CAD build for the part. Positions are in the model's coordinates, mm. A direction names the side the tool comes from. Round coordinates to 2 decimals unless told otherwise and drop trailing zeros. Order: outer loops, then holes, each group sorted by start corner. A loop starts at its lowest first (then second) coordinate and runs counter-clockwise, first axis right, second up. Notation, with made-up numbers: M 51,15.5 L 68,15.5 A20 ccw 68,24.5 Z; hole C 7,26 d6. An arc over 180 degrees is marked long. Put each result on its own line as item: value.
```python
from build123d import *

# Parameters (mm, degrees)
F0_R     = 2
F1_DEPTH = 5
F2_R     = 3
F3_DEPTH = 10
F4_R     = 1.3
F5_DEPTH = 10


with BuildPart() as f1:
    # F0 (on Front) → F1 (new body)
    with BuildSketch(Plane.XZ):
        with BuildLine():
            Line((-2, 3.338963), (-2, 12.338963))
            ThreePointArc((-2, 12.338963), (-10.825318, 6.25), (-11.685855, -4.437431))
            Line((-11.685855, -4.437431), (-3.891627, 0.062569))
            Line((-3.891627, 0.062569), (-1.891627, -3.401532))
            Line((-1.891627, -3.401532), (-9.685855, -7.901532))
            ThreePointArc((-9.685855, -7.901532), (0, -12.5), (9.685855, -7.901532))
            Line((9.685855, -7.901532), (1.891627, -3.401532))
            Line((1.891627, -3.401532), (3.891627, 0.062569))
            Line((3.891627, 0.062569), (11.685855, -4.437431))
            ThreePointArc((11.685855, -4.437431), (10.825318, 6.25), (2, 12.338963))
            Line((2, 12.338963), (2, 3.338963))
            Line((2, 3.338963), (-2, 3.338963))
        make_face()
        Circle(F0_R, mode=Mode.SUBTRACT)
    extrude(amount=F1_DEPTH)

    # F2 (on face) → F3 (join)
    with BuildSketch(Plane.XZ.offset(5)):
        with Locations((7.794229, 4.5)):
            Circle(F2_R)
        with Locations((-7.794229, 4.5)):
            Circle(F2_R)
        with Locations((0, -9)):
            Circle(F2_R)
    extrude(amount=F3_DEPTH)

    # F4 (on face) → F5 (cut)
    with BuildSketch(Plane.XZ.offset(15)):
        with Locations((0, -9)):
            Circle(F4_R)
        with Locations((7.794229, 4.5)):
            Circle(F4_R)
        with Locations((-7.794229, 4.5)):
            Circle(F4_R)
    extrude(amount=-F5_DEPTH, mode=Mode.SUBTRACT)


solid = f1.part
```
Item 1: Band-saw the part on D-D on y = -2. Give the cut face in (x, z).
Answers below:
outline: M -11.69,-4.44 L -3.89,0.06 L -1.89,-3.4 L -9.69,-7.9 A12.5 ccw 9.69,-7.9 L 1.89,-3.4 L 3.89,0.06 L 11.69,-4.44 A12.5 ccw 2,12.34 L 2,3.34 L -2,3.34 L -2,12.34 A12.5 ccw Z; hole C 0,0 d4
Item 2: Tool access for faces 4 (the flat face through (-7, -15, 3)), 5 (the flat face through (-2.906, -2.465, -1.645)), 6 (the cylindrical face through (0, -10, -6)): list every direction of +Z, -Z, +X, -X, +Y, -Y with a clear straight run to the whole face (end or side of a thin tool).
Answers below:
face 4: +Z, -Z, +X, -X, -Y
face 5: +Y, -Y
face 6: -Y
Item 3: Probe line 1 along Z through (x, y) = (0, -12); line 2 along Y through (x, z) = (-4, -8.25); line 3 along Z through (x, y) = (-0.5, -6.5). List the from-to ranges inside material, lowest first. Write a range as [from, to].
Answers below:
line 1: [-12, -10.3], [-7.7, -6]
line 2: [-5, 0]
line 3: [-11.96, -10.2], [-7.8, -6.04]
Item 4: Mould opens along Z. For faces 1 (the cylindrical face through (-10.75, -2.46, 6.38)), 2 (the flat face through (0, -5, -9)), 3 (the flat face through (3, -5, 0)) say: pulls with the +Z half, pulls with the -Z half, needs draft (parallel to the pull), parting line crosses it, or undercut.
Answers below:
face 1: parting line crosses it
face 2: undercut
face 3: needs draft
Item 5: Band-saw the part on A-A on x = 0. Give the cut face in (y, z), and give its area (3 significant figures).
Answers below:
outline: M -15,-12 L -5,-12 L -5,-12.5 L 0,-12.5 L 0,-2 L -5,-2 L -5,-6 L -15,-6 L -15,-7.7 L -5,-7.7 L -5,-10.3 L -15,-10.3 Z; M -5,2 L 0,2 L 0,3.34 L -5,3.34 Z
area: 93.2 mm²
Item 6: Pin check, flat tips, straight feed: P1, Ø4, axis at x = -3.5, y = -5, coming from the -Z side; P2, Ø5, axis at x = 6.5, y = -6, coming from the -Z side; P3, Ø4, axis at y = -4.5, z = -7, coming from the +X side. Stop position of each tip, or through.
Answers below:
P1: z = -12.41
P2: z = -11.77
P3: x = 9.69
Item 7: Band-saw the part on B-B on z = -2.75. Give the cut face in (x, y), and give its area (3 significant figures).
Answers below:
outline: M -12.19,-5 L -8.76,-5 L -8.76,0 L -12.19,0 Z; M -2.27,-5 L 2.27,-5 L 2.27,0 L -2.27,0 Z; M 8.76,-5 L 12.19,-5 L 12.19,0 L 8.76,0 Z
area: 57.0 mm²
Item 8: Band-saw the part on C-C on y = -8. Give the cut face in (x, z), and give its area (3 significant figures).
Answers below:
outline: C -7.79,4.5 d6; C 0,-9 d6; C 7.79,4.5 d6; hole C -7.79,4.5 d2.6; hole C 0,-9 d2.6; hole C 7.79,4.5 d2.6
area: 68.9 mm²
